Geometry check sheet. Reference: the model listing, model coordinates, mm. Round coordinates to 2 decimals unless told otherwise and drop trailing zeros. Use one line per item in the form item = value.
from build123d import *


with BuildPart() as f3:
    # F0 (on Top) → F3 section 0
    with BuildSketch(Plane.XY):
        with BuildLine():
            ThreePointArc((11.91593, 3.907013), (10.670413, 4.41983), (11.18851, 5.66316))
            ThreePointArc((11.18851, 5.66316), (11.63221, 11.63221), (5.66316, 11.18851))
            ThreePointArc((5.66316, 11.18851), (4.41983, 10.670413), (3.907013, 11.91593))
            ThreePointArc((3.907013, 11.91593), (0, 16.450429), (-3.907013, 11.91593))
            ThreePointArc((-3.907013, 11.91593), (-4.41983, 10.670413), (-5.66316, 11.18851))
            ThreePointArc((-5.66316, 11.18851), (-11.63221, 11.63221), (-11.18851, 5.66316))
            ThreePointArc((-11.18851, 5.66316), (-10.670413, 4.41983), (-11.91593, 3.907013))
            ThreePointArc((-11.91593, 3.907013), (-16.450429, 0), (-11.91593, -3.907013))
            ThreePointArc((-11.91593, -3.907013), (-10.670413, -4.41983), (-11.18851, -5.66316))
            ThreePointArc((-11.18851, -5.66316), (-11.63221, -11.63221), (-5.66316, -11.18851))
            ThreePointArc((-5.66316, -11.18851), (-4.41983, -10.670413), (-3.907013, -11.91593))
            ThreePointArc((-3.907013, -11.91593), (0, -16.450429), (3.907013, -11.91593))
            ThreePointArc((3.907013, -11.91593), (4.41983, -10.670413), (5.66316, -11.18851))
            ThreePointArc((5.66316, -11.18851), (11.63221, -11.63221), (11.18851, -5.66316))
            ThreePointArc((11.18851, -5.66316), (10.670413, -4.41983), (11.91593, -3.907013))
            ThreePointArc((11.91593, -3.907013), (16.450429, 0), (11.91593, 3.907013))
        make_face()
    # F2 (on offset) → F3 section 1
    with BuildSketch(Plane.XY.offset(100)):
        with BuildLine():
            ThreePointArc((24.202745, 6.351012), (19.955006, 8.265634), (21.604769, 12.623082))
            ThreePointArc((21.604769, 12.623082), (22.203759, 22.203759), (12.623082, 21.604769))
            ThreePointArc((12.623082, 21.604769), (8.265634, 19.955006), (6.351012, 24.202745))
            ThreePointArc((6.351012, 24.202745), (0, 31.400857), (-6.351012, 24.202745))
            ThreePointArc((-6.351012, 24.202745), (-8.265634, 19.955006), (-12.623082, 21.604769))
            ThreePointArc((-12.623082, 21.604769), (-22.203759, 22.203759), (-21.604769, 12.623082))
            ThreePointArc((-21.604769, 12.623082), (-19.955006, 8.265634), (-24.202745, 6.351012))
            ThreePointArc((-24.202745, 6.351012), (-31.400857, 0), (-24.202745, -6.351012))
            ThreePointArc((-24.202745, -6.351012), (-19.955006, -8.265634), (-21.604769, -12.623082))
            ThreePointArc((-21.604769, -12.623082), (-22.203759, -22.203759), (-12.623082, -21.604769))
            ThreePointArc((-12.623082, -21.604769), (-8.265634, -19.955006), (-6.351012, -24.202745))
            ThreePointArc((-6.351012, -24.202745), (0, -31.400857), (6.351012, -24.202745))
            ThreePointArc((6.351012, -24.202745), (8.265634, -19.955006), (12.623082, -21.604769))
            ThreePointArc((12.623082, -21.604769), (22.203759, -22.203759), (21.604769, -12.623082))
            ThreePointArc((21.604769, -12.623082), (19.955006, -8.265634), (24.202745, -6.351012))
            ThreePointArc((24.202745, -6.351012), (31.400857, 0), (24.202745, 6.351012))
        make_face()
    loft()


solid = f3.part
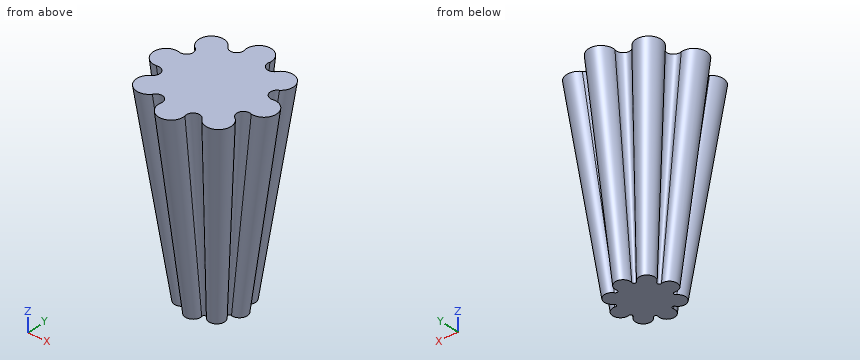
1. Section check A-A (y = -23). Count the separate pieces of the cut face and the enclosed holes in it, then the cut area to 3 significant figures.
Return value:
separate_pieces = 3
enclosed_holes = 0
area = 648 mm2
2. Gauge pin test, flat ends, axial feed: pin 1 (8 mm diameter, centred on x = 1, z = 18, fed in from -Y); pin 2 (1 mm diameter, centred on y = 0.5, z = 55, fed in from -X); pin 3 (5 mm diameter, centred on y = 13, z = 73, fed in from -X). Record the tip position at first contact, or that the pin passes through.
Return value:
pin_1 = -19.72
pin_2 = -24.73
pin_3 = -21.19
3. Material ranges on line 1 along X through (y, z) = (-15, 26.5); line 2 along X through (y, z) = (14, 32); line 3 along X through (y, z) = (19, 32), recorded low to high.
Return value:
line_1 = -13.75 to -8.62, -4.5 to 4.5, 8.62 to 13.75
line_2 = -15.79 to -7.52, -5.11 to 5.11, 7.52 to 15.79
line_3 = -4.02 to 4.02
